Can you work these out from the model? Positions are in its coordinate system, mm. Face numbers are marked on the shaded views. Give positions to 0.01 mm unless a question says otherwise; leave off trailing zeros. Order: outer loops, then holes, each group sorted by start corner. A loop starts at its lowest first (then second) coordinate and runs counter-clockwise, first axis right, second up.
Item 1: I want a section at A-A, the plane x = 0. Write out the boundary of the cut face in (y, z).
Item 2: I want a section at C-C, the plane z = 1.4. Write out the boundary of the cut face in (x, y), then the cut area to 3 significant figures.
Item 3: If I drill on line 1 along Y through (x, z) = (0, 2); line 2 along X through (y, z) = (-2, 1); line 3 along X through (y, z) = (0, 1.2), over which ranges is the centre line in solid material (lowest first)?
Item 4: If we mould it in two halves opening along X, with no side actions, what happens to the marked faces 1, 2 and 3? For each: +X half, -X half, draft (parallel to the pull), parting line (faces both ways), or undercut.
Item 5: I'm going to push flat-ended pins straight in: pin 1 Ø4 at (x, y) = (2, 0.5) entering from -Z; pin 2 Ø1 at (y, z) = (-3, 1.5) entering from -X. Where does each tip first touch, or does it pass through?
Autodesk Fusion 360 part; units mm, degrees
sketch "Sketch2" plane through (0, 0, 0) normal (0, 1, 0) x (1, 0, 0)
  line L0 (0, -5.5) -> (0, 3.2)
  line L1 (0, 0) -> (4.9, 0) construction
  line L2 (4.9, 0) -> (4.9, -2.15)
  line L3 (4.9, 0) -> (7.8, 0)
  line L4 (7.8, 0) -> (7.8, -0.5)
  line L5 (4.9, -2.15) -> (5.5, -2.15)
  line L6 (5.5, -2.15) -> (5.5, -1.9)
  line L7 (5.5, -1.9) -> (6.5, -1.9)
  line L8 (6.5, -1.9) -> (7.8, -0.5)
  dimension "d3" = 4.9
  dimension "d4" = 2.15
  dimension "d5" = 2.9
  dimension "d6" = 0.5
  dimension "d7" = 0.6
  dimension "d8" = 1.9
  dimension "d9" = 1.6
revolve "Revolve1" add sketch "Sketch2" angle 360 about axis through (0, 0, 5.5) along (0, 0, -1)
equation "d3 = ( 9.8 / 2 ) * 1 mm"
equation "d5 = ( 15.6 / 2 ) * 1 mm - 4.9 mm"
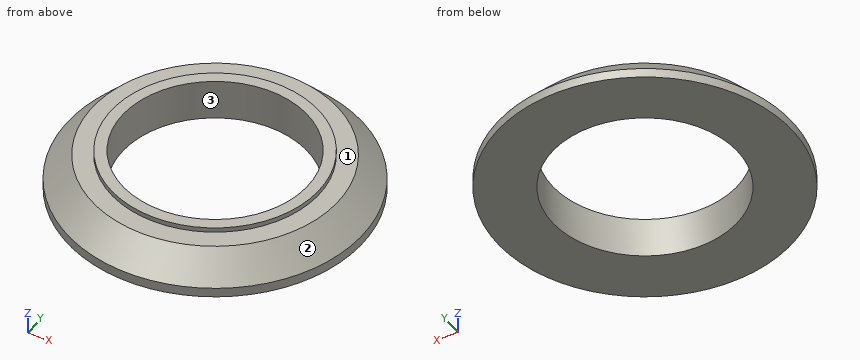
Results list:
1. outline: (-7.8, 0) - (-4.9, 0) - (-4.9, 2.15) - (-5.5, 2.15) - (-5.5, 1.9) - (-6.5, 1.9) - (-7.8, 0.5) - close; (4.9, 0) - (7.8, 0) - (7.8, 0.5) - (6.5, 1.9) - (5.5, 1.9) - (5.5, 2.15) - (4.9, 2.15) - close
2. outline: circle Ø13.93 at (0, 0); hole circle Ø9.8 at (0, 0)
2. area: 76.9 mm2
3. line 1: y = -5.5 to -4.9, 4.9 to 5.5
3. line 2: x = -7.06 to -4.47, 4.47 to 7.06
3. line 3: x = -7.15 to -4.9, 4.9 to 7.15
4. face 1: draft
4. face 2: parting line
4. face 3: undercut
5. pin 1: passes through
5. pin 2: stops at x = -6.74
